For this review, take the finished solid that the model builds, in its own axes (mm). Face numbers are marked on the shaded views. A direction names the side the tool comes from. Round coordinates to 2 decimals unless told otherwise and drop trailing zeros. Order: outer loops, then holes, each group sorted by start corner. A loop starts at its lowest first (then second) coordinate and runs counter-clockwise, first axis right, second up. Notation, with made-up numbers: M -15,-21 L 25,-21 A24 ccw 25,6 Z; hole C -36,56 d3. An arc over 180 degrees is marked long. Use a Markdown table: item, result.
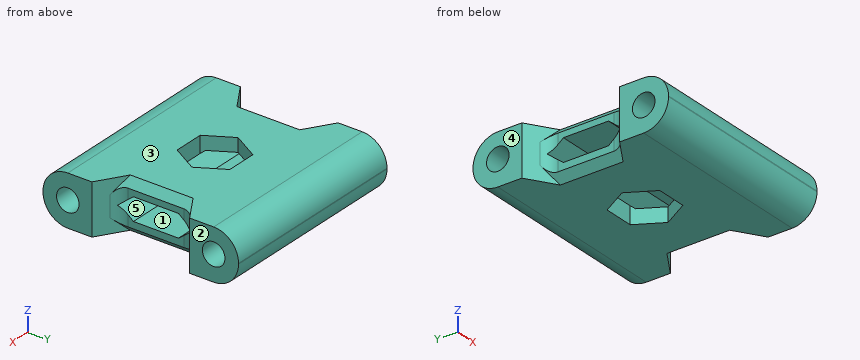
from build123d import *

# Parameters (mm, degrees)
F1_DEPTH = 1.675
F2_SIZE  = 0.5
F3_R     = 1.65
F4_R     = 1
F5_R     = 0.75
F6_DEPTH = 13.001


with BuildPart() as f1:
    # F0 (on Top) → F1 (new body, symmetric)
    with BuildSketch(Plane.XY):
        Polygon((6.5, 6.5), (-6.5, 6.5), (-6.5, 3.25), (-5.168492, 2.405253), (-5.168492, -2.405253), (-6.5, -3.25), (-6.5, -6.5), (6.5, -6.5), (6.5, -3.25), (5.168492, -2.405253), (5.168492, 2.405253), (6.5, 3.25), align=None)
        Polygon((-2.021299, 0), (-1.01065, 1.750496), (1.01065, 1.750496), (2.021299, 0), (1.01065, -1.750496), (-1.01065, -1.750496), align=None, mode=Mode.SUBTRACT)
    extrude(amount=F1_DEPTH, both=True)

    # F2
    f2_edges = [f1.edges().sort_by_distance(p)[0] for p in [
        (-5.168492, 0, 1.675),
        (5.168492, 0, 1.675),
        (-5.168492, 0, -1.675),
        (5.168492, 0, -1.675),
    ]]
    chamfer(f2_edges, length=F2_SIZE)

    # F3
    f3_edges = [f1.edges().sort_by_distance(p)[0] for p in [
        (0, 6.5, 1.675),
        (0, 6.5, -1.675),
        (0, -6.5, 1.675),
        (0, -6.5, -1.675),
    ]]
    fillet(f3_edges, radius=F3_R)

    # F4
    f4_edges = [f1.edges().sort_by_distance(p)[0] for p in [
        (5.168492, 2.405253, 0),
        (5.168492, -2.405253, 0),
        (-5.168492, -2.405253, 0),
        (-5.168492, 2.405253, 0),
    ]]
    fillet(f4_edges, radius=F4_R)

    # F5 (on face) → F6 (cut, through all)
    with BuildSketch(Plane.YZ.offset(6.5)):
        with Locations((-4.85, 0.025)):
            Circle(F5_R)
        with Locations((4.85, 0.025)):
            Circle(F5_R)
        Polygon((-1.499787, 0.775), (-2.422007, 0.025), (-1.499787, -0.725), (1.499787, -0.725), (2.442251, 0.025), (1.499787, 0.775), align=None)
    extrude(amount=-F6_DEPTH, mode=Mode.SUBTRACT)


solid = f1.part
Q1. Wall thickness on line 1 along X through (y, z) = (1.5, -1.1); line 2 along Y through (x, z) = (4.5, -0.2); line 3 along Z through (x, y) = (-1.75, 1.75) (3 decimals): over which ranges is each line inside the solid? List them lowest first. Write a range as [from, to].
Determined:
| item | result |
|---|---|
| line 1 | x = [-5.17, -1.16], [1.16, 5.17] |
| line 2 | y = [-6.49, -5.57], [-4.13, -2.15], [2.16, 4.13], [5.57, 6.49] |
| line 3 | z = [-1.675, -0.526], [0.576, 1.675] |
Q2. Draft analysis for pull direction Z (two halves, no side actions). For the marked faces 1, 2 and 3, state which applies: pulls with the +Z half, pulls with the -Z half, needs draft (parallel to the pull), parting line crosses it, or undercut.
Determined:
| item | result |
|---|---|
| face 1 | undercut |
| face 2 | needs draft |
| face 3 | pulls with the +Z half |
Q3. Add section C-C (y = 0.25). Write out the cut boundary in (x, z) (1 decimal), then the cut area to 3 significant figures.
Determined:
| item | result |
|---|---|
| outline | M -5.2,-1.2 L -4.7,-1.7 L -1.9,-1.7 L -1.9,-0.7 L -5.2,-0.7 Z; M -5.2,0.8 L -1.9,0.8 L -1.9,1.7 L -4.7,1.7 L -5.2,1.2 Z; M 1.9,-1.7 L 4.7,-1.7 L 5.2,-1.2 L 5.2,-0.7 L 1.9,-0.7 Z; M 1.9,0.8 L 5.2,0.8 L 5.2,1.2 L 4.7,1.7 L 1.9,1.7 Z |
| area | 11.7 mm^2 |
Q4. Clearance check with flat-ended pins moving along their axes: pin 1 (0.8 mm diameter, centred on y = 0, z = -0.5, fed in from +X); pin 2 (0.6 mm diameter, centred on x = 0, z = -1, fed in from -Y); pin 3 (1.2 mm diameter, centred on x = -0.5, z = 1, fed in from -Y). State where each tip first meets the part, or that it passes through.
Determined:
| item | result |
|---|---|
| pin 1 | stops at x = 5.17 |
| pin 2 | stops at y = -6.36 |
| pin 3 | stops at y = -6.46 |
Q5. Add section D-D (z = -1.4). Write out the cut boundary in (x, y), then the cut area to 3 significant figures.
Determined:
| item | result |
|---|---|
| outline | M -6.5,-5.76 L 6.5,-5.76 L 6.5,-3.25 L 4.94,-2.26 L 4.94,2.26 L 6.5,3.25 L 6.5,5.76 L -6.5,5.76 L -6.5,3.25 L -4.94,2.26 L -4.94,-2.26 L -6.5,-3.25 Z; hole M -2.02,0 L -1.01,-1.75 L 1.01,-1.75 L 2.02,0 L 1.01,1.75 L -1.01,1.75 Z |
| area | 122 mm^2 |
Q6. Machinability: for the marked faces 4 and 5, which of the approach directions +Z, -Z, +X, -X, +Y, -Y give a long, thin tool a straight path to every point of the face, cutting with its end or side? Answer none if there is none.
Determined:
| item | result |
|---|---|
| face 4 | +Z, -Z, -X, +Y, -Y |
| face 5 | +X, -X |
Q7. Add section A-A (y = -4.25). Write out the cut boundary in (x, z) (3 decimals).
Determined:
| item | result |
|---|---|
| outline | M -6.5,-1.675 L 6.5,-1.675 L 6.5,-0.425 L -6.5,-0.425 Z; M -6.5,0.475 L 6.5,0.475 L 6.5,1.675 L -6.5,1.675 Z |
Q8. Add section B-B (x = 2.5). Write out the cut boundary in (y, z) (3 decimals).
Determined:
| item | result |
|---|---|
| outline | M -6.5,-0.025 A1.65 ccw -4.85,-1.675 L 4.85,-1.675 A1.65 ccw 6.5,-0.025 L 6.5,0.025 A1.65 ccw 4.85,1.675 L -4.85,1.675 A1.65 ccw -6.5,0.025 Z; hole C -4.85,0.025 d1.5; hole M -2.422,0.025 L -1.5,-0.725 L 1.5,-0.725 L 2.442,0.025 L 1.5,0.775 L -1.5,0.775 Z; hole C 4.85,0.025 d1.5 |
